```python
from build123d import *

# Parameters (mm, degrees)
F1_DEPTH = 3


with BuildPart() as f1:
    # F0 (on Front) → F1 (new body)
    with BuildSketch(Plane.XZ):
        with BuildLine():
            ThreePointArc((19.64988, 1.433678), (15.323457, 4.878104), (10.650251, 7.834987))
            ThreePointArc((10.650251, 7.834987), (6.630714, 8.466829), (2.786874, 7.132363))
            ThreePointArc((2.786874, 7.132363), (-0.723137, 8.153352), (-4.378306, 8.104974))
            ThreePointArc((-4.378306, 8.104974), (-6.665865, 7.454354), (-8.461449, 5.894833))
            ThreePointArc((-8.461449, 5.894833), (-11.303445, 3.882664), (-14.034172, 1.7219))
            ThreePointArc((-14.034172, 1.7219), (-16.241362, 0.362004), (-18.739592, -0.33071))
            ThreePointArc((-18.739592, -0.33071), (-20.184903, 0.439819), (-20.795666, 1.959558))
            ThreePointArc((-20.795666, 1.959558), (-20.5849, 2.899405), (-19.829269, 3.496695))
            ThreePointArc((-19.829269, 3.496695), (-18.935867, 3.784112), (-18.032324, 4.037856))
            ThreePointArc((-18.032324, 4.037856), (-17.638426, 4.218128), (-17.404594, 4.582786))
            ThreePointArc((-17.404594, 4.582786), (-18.437288, 5.04708), (-19.567223, 5.119697))
            ThreePointArc((-19.567223, 5.119697), (-20.879767, 4.775386), (-22.018788, 4.037856))
            ThreePointArc((-22.018788, 4.037856), (-23.375832, 2.054301), (-23.672102, -0.33071))
            ThreePointArc((-23.672102, -0.33071), (-23.000152, -1.878598), (-21.816935, -3.081708))
            ThreePointArc((-21.816935, -3.081708), (-20.983966, -3.693037), (-20.110425, -4.244841))
            Line((-20.110425, -4.244841), (-20.10519, -4.36016))
            Line((-20.10519, -4.36016), (-20.10519, -17.453194))
            Line((-20.10519, -17.453194), (-18.60519, -17.453194))
            Line((-18.60519, -17.453194), (-18.60519, -5.012271))
            ThreePointArc((-18.60519, -5.012271), (-18.322698, -5.133071), (-18.037762, -5.247988))
            Line((-18.037762, -5.247988), (-18.032324, -17.453194))
            Line((-18.032324, -17.453194), (-16.532324, -17.453194))
            Line((-16.532324, -17.453194), (-16.532324, -5.745979))
            ThreePointArc((-16.532324, -5.745979), (-16.219609, -5.827508), (-15.90519, -5.902199))
            Line((-15.90519, -5.902199), (-15.90519, -17.453194))
            Line((-15.90519, -17.453194), (-14.40519, -17.453194))
            Line((-14.40519, -17.453194), (-14.40519, -6.161144))
            ThreePointArc((-14.40519, -6.161144), (-14.189632, -6.185442), (-13.973741, -6.206582))
            Line((-13.973741, -6.206582), (-13.968729, -17.453194))
            Line((-13.968729, -17.453194), (-12.468729, -17.453194))
            Line((-12.468729, -17.453194), (-12.468729, -6.355174))
            ThreePointArc((-12.468729, -6.355174), (-12.08716, -6.383263), (-11.70519, -6.405258))
            Line((-11.70519, -6.405258), (-11.70519, -17.453194))
            Line((-11.70519, -17.453194), (-10.20519, -17.453194))
            Line((-10.20519, -17.453194), (-10.20519, -6.432613))
            ThreePointArc((-10.20519, -6.432613), (-9.869726, -6.425881), (-9.53439, -6.414452))
            Line((-9.53439, -6.414452), (-9.52947, -17.453194))
            Line((-9.52947, -17.453194), (-8.02947, -17.453194))
            Line((-8.02947, -17.453194), (-8.02947, -6.305079))
            ThreePointArc((-8.02947, -6.305079), (-7.767164, -6.276231), (-7.50519, -6.244497))
            Line((-7.50519, -6.244497), (-7.50519, -17.453194))
            Line((-7.50519, -17.453194), (-6.00519, -17.453194))
            Line((-6.00519, -17.453194), (-6.00519, -6.044151))
            Line((-6.00519, -6.044151), (-6.006557, -6.006161))
            ThreePointArc((-6.006557, -6.006161), (-5.736134, -5.952714), (-5.466344, -5.89616))
            Line((-5.466344, -5.89616), (-5.461194, -17.453194))
            Line((-5.461194, -17.453194), (-3.961194, -17.453194))
            Line((-3.961194, -17.453194), (-3.961194, -5.52024))
            ThreePointArc((-3.961194, -5.52024), (-3.632846, -5.432887), (-3.30519, -5.342972))
            Line((-3.30519, -5.342972), (-3.30519, -17.453194))
            Line((-3.30519, -17.453194), (-1.80519, -17.453194))
            Line((-1.80519, -17.453194), (-1.80519, -4.895811))
            ThreePointArc((-1.80519, -4.895811), (-1.486897, -4.793308), (-1.169401, -4.688361))
            Line((-1.169401, -4.688361), (-1.163963, -17.453194))
            Line((-1.163963, -17.453194), (0.336037, -17.453194))
            Line((0.336037, -17.453194), (0.336037, -4.153387))
            ThreePointArc((0.336037, -4.153387), (0.623788, -4.043977), (0.910758, -3.932534))
            Line((0.910758, -3.932534), (0.89481, -4.038423))
            Line((0.89481, -4.038423), (0.89481, -17.453194))
            Line((0.89481, -17.453194), (2.39481, -17.453194))
            Line((2.39481, -17.453194), (2.39481, -3.318312))
            ThreePointArc((2.39481, -3.318312), (2.591489, -3.232046), (2.78774, -3.14481))
            Line((2.78774, -3.14481), (2.786874, -17.453194))
            Line((2.786874, -17.453194), (4.286874, -17.453194))
            Line((4.286874, -17.453194), (4.286874, -3.791388))
            ThreePointArc((4.286874, -3.791388), (4.50534, -3.931658), (4.726803, -4.067149))
            Line((4.726803, -4.067149), (4.726803, -17.453194))
            Line((4.726803, -17.453194), (6.226803, -17.453194))
            Line((6.226803, -17.453194), (6.226803, -4.824973))
            ThreePointArc((6.226803, -4.824973), (6.500619, -4.935953), (6.777095, -5.040129))
            Line((6.777095, -5.040129), (6.777095, -17.453194))
            Line((6.777095, -17.453194), (8.277095, -17.453194))
            Line((8.277095, -17.453194), (8.277095, -5.475662))
            ThreePointArc((8.277095, -5.475662), (8.588473, -5.54004), (8.901453, -5.596111))
            Line((8.901453, -5.596111), (8.901453, -17.453194))
            Line((8.901453, -17.453194), (10.401453, -17.453194))
            Line((10.401453, -17.453194), (10.401453, -5.844886))
            ThreePointArc((10.401453, -5.844886), (10.683933, -5.897254), (10.96692, -5.946817))
            Line((10.96692, -5.946817), (10.972047, -17.453194))
            Line((10.972047, -17.453194), (12.472047, -17.453194))
            Line((12.472047, -17.453194), (12.472047, -6.162236))
            ThreePointArc((12.472047, -6.162236), (12.769688, -6.195327), (13.067656, -6.225338))
            Line((13.067656, -6.225338), (13.073482, -17.453194))
            Line((13.073482, -17.453194), (14.584494, -17.453194))
            Line((14.584494, -17.453194), (14.584494, -6.330084))
            ThreePointArc((14.584494, -6.330084), (14.88197, -6.341257), (15.179546, -6.349371))
            Line((15.179546, -6.349371), (15.184494, -17.453194))
            Line((15.184494, -17.453194), (16.684494, -17.453194))
            Line((16.684494, -17.453194), (16.684494, -6.343539))
            ThreePointArc((16.684494, -6.343539), (16.980227, -6.33319), (17.27584, -6.319818))
            Line((17.27584, -6.319818), (17.27584, -6.356424))
            Line((17.27584, -6.356424), (17.27584, -17.453194))
            Line((17.27584, -17.453194), (18.77584, -17.453194))
            Line((18.77584, -17.453194), (18.77584, -6.205151))
            ThreePointArc((18.77584, -6.205151), (19.113283, -6.168516), (19.450272, -6.127927))
            Line((19.450272, -6.127927), (19.455319, -17.453194))
            Line((19.455319, -17.453194), (20.955319, -17.453194))
            Line((20.955319, -17.453194), (20.955319, -5.91936))
            ThreePointArc((20.955319, -5.91936), (21.263829, -5.876265), (21.571221, -5.82581))
            Line((21.571221, -5.82581), (21.571221, -17.453194))
            Line((21.571221, -17.453194), (23.071221, -17.453194))
            Line((23.071221, -17.453194), (23.071221, -5.468547))
            Line((23.071221, -5.468547), (23.425881, -5.329391))
            Line((23.425881, -5.329391), (23.425881, -17.453194))
            Line((23.425881, -17.453194), (24.779715, -17.453194))
            Line((24.779715, -17.453194), (24.779715, -4.81928))
            Line((24.779715, -4.81928), (25.144875, -4.61932))
            Line((25.144875, -4.61932), (25.144875, -17.453194))
            Line((25.144875, -17.453194), (26.461203, -17.453194))
            Line((26.461203, -17.453194), (26.461203, -4.36016))
            Line((26.461203, -4.36016), (26.461203, -3.884922))
            ThreePointArc((26.461203, -3.884922), (26.789065, -3.662423), (27.110012, -3.430062))
            ThreePointArc((27.110012, -3.430062), (28.749864, -1.609204), (29.219028, 0.7959))
            ThreePointArc((29.219028, 0.7959), (28.672922, 2.715777), (27.348137, 4.208795))
            ThreePointArc((27.348137, 4.208795), (26.308789, 4.900953), (25.106104, 5.236921))
            ThreePointArc((25.106104, 5.236921), (23.892424, 5.002762), (22.945076, 4.208795))
            ThreePointArc((22.945076, 4.208795), (23.790754, 3.790745), (24.726035, 3.667505))
            ThreePointArc((24.726035, 3.667505), (25.403757, 3.496758), (26.01371, 3.155556))
            ThreePointArc((26.01371, 3.155556), (26.358297, 2.455561), (26.280997, 1.679185))
            ThreePointArc((26.280997, 1.679185), (25.668609, 0.851297), (24.878269, 0.19116))
            ThreePointArc((24.878269, 0.19116), (23.775899, -0.249398), (22.591121, -0.174478))
            ThreePointArc((22.591121, -0.174478), (21.034715, 0.472702), (19.64988, 1.433678))
        make_face()
    extrude(amount=F1_DEPTH)


solid = f1.part
```
Geometry check sheet. Reference: the model listing, model coordinates, mm. A direction names the side the tool comes from. Coordinates: 2 decimals unless noted, no trailing zeros. Write each loop counter-clockwise with the first axis right and the second up, starting at its lowest first coordinate (ties: lowest second). Pieces come first, ordered by that corner, then holes. Notation, with made-up numbers: M 34.5,18.25 L 89.5,18.25 A29 ccw 89.5,43.25 Z; hole C 0,25.5 d1. An arc over 180 degrees is marked long. One line per item, written item: value. Start each with the question number.
(1) Sectioned sample at D-D, the plane x = 18. Enter the section's corners in (y, z).
(2) Sectioned sample at A-A, the plane z = -10.25. State how many separate pieces and enclosed holes the cut face has, and give its area (3 significant figures).
(3) Sectioned sample at B-B, the plane x = 3.5. Enter the section's corners in (y, z).
(4) Depth check by flat-ended pin: pin 1 (1.5 mm diameter, centred on y = -1, z = -10.5, fed in from -X); pin 2 (0.9 mm diameter, centred on y = -1, z = -12, fed in from +X). Enter the tip coordinate at first touch or a pass-through.
(5) Release check for a two-part mould opening along X. For faces 1 (the face through (-18.422, -1.479, 5.043)), 2 (the face through (2, -1, -17.453)), 3 (the face through (26.325, -1.479, 4.894)) record: released by +X, released by -X, zero draft, split by the parting line, or undercut.
(6) Tool access check on faces 4 (the face through (-20.169, -1.479, 0.422)), 5 (the face through (-11, -1, -17.453)), 6 (the face through (10.401, -1, -12)). Record the directions out of +Z, -Z, +X, -X, +Y, -Y that give a thin tool (end or side, any length) a straight path to the whole face; none if there is none.
(7) Scan lines: line 1 along X through (y, z) = (-2.55, 2.25); line 2 along X through (y, z) = (-1.75, 2); line 3 along Z through (x, y) = (20.5, -2.6). Record each from-to range of solid material in increasing order. Write a range as [from, to].
Filled sheet:
1. outline: M -3,-17.45 L 0,-17.45 L 0,2.84 L -3,2.84 Z
2. separate pieces: 23
2. enclosed holes: 0
2. area: 103 mm²
3. outline: M -3,-17.45 L 0,-17.45 L 0,7.55 L -3,7.55 Z
4. pin 1: x = -20.11
4. pin 2: x = 26.46
5. face 1: undercut
5. face 2: zero draft
5. face 3: released by +X
6. face 4: +Y, -Y
6. face 5: -Z, +X, -X, +Y, -Y
6. face 6: -Z, +Y, -Y
7. line 1: [-23.3, -20.8], [-13.39, 18.71], [26.38, 28.89]
7. line 2: [-23.4, -20.8], [-13.7, 19], [26.37, 28.99]
7. line 3: [-17.45, 0.79]
